The model under review builds one solid part; all positions refer to its coordinate system, in mm. Face numbers are marked on the shaded views. A direction names the side the tool comes from. Coordinates: 2 decimals unless noted, no trailing zeros. Write each loop counter-clockwise with the first axis right and the second up, starting at its lowest first coordinate (ties: lowest second). Pieces come first, ordered by that corner, then holes. Notation, with made-up numbers: M 19.5,49.5 L 38.5,49.5 A23 cw 38.5,88.5 Z; hole C 40.25,66.25 d11. An arc over 180 degrees is marked long. Answer as a JSON object with one key per item and string values.
```python
from build123d import *

# Parameters (mm, degrees)
BOSS_EXTRUDE1_DEPTH = 1013.2


with BuildPart() as part:
    # Sketch1 → Boss-Extrude1 (new body)
    with BuildSketch(Plane.XY):
        Polygon((1221.8, 1649.71), (2235, 1649.71), (2235, 0), (0, 0), (0, 1053.44), align=None)
        Polygon((2.5, 1051.878238321), (1222.377482381, 1647.21), (2232.5, 1647.21), (2232.5, 2.5), (2.5, 2.5), align=None, mode=Mode.SUBTRACT)
    extrude(amount=BOSS_EXTRUDE1_DEPTH)


solid = part.part
```
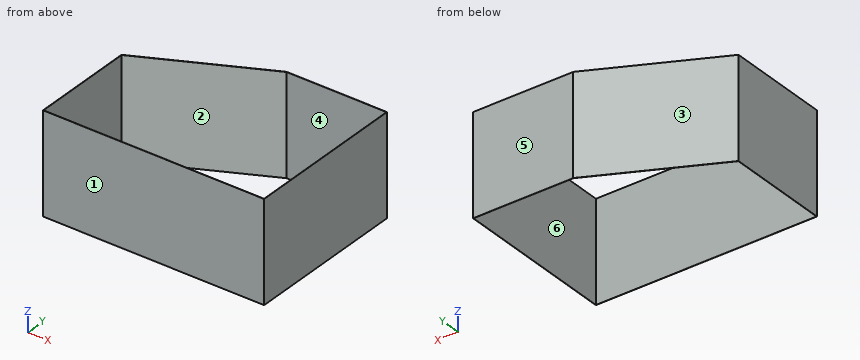
(1) Draft analysis for pull direction X (two halves, no side actions). For the marked faces 1, 2, 3 and 4, state which applies: released by +X, released by -X, zero draft, split by the parting line, or undercut.
Results list:
{"face 1": "zero draft", "face 2": "undercut", "face 3": "released by -X", "face 4": "undercut"}
(2) Add section C-C on z = 730. Give the boundary of the cut face in (x, y), and give its area (3 significant figures).
Results list:
{"outline": "M 0,0 L 2235,0 L 2235,1649.71 L 1221.8,1649.71 L 0,1053.44 Z; hole M 2.5,2.5 L 2232.5,2.5 L 2232.5,1647.21 L 1222.38,1647.21 L 2.5,1051.88 Z", "area": "18,300 mm²"}
(3) Add section A-A on x = 1362. Give the boundary of the cut face in (y, z).
Results list:
{"outline": "M 0,0 L 2.5,0 L 2.5,1013.2 L 0,1013.2 Z; M 1647.21,0 L 1649.71,0 L 1649.71,1013.2 L 1647.21,1013.2 Z"}
(4) For pin 1 Ø12 at (x, z) = (329, 668.5) entering from +Y; pin 2 Ø5 at (x, z) = (974, 269) entering from +Y; pin 3 Ø3 at (y, z) = (394, 376) entering from -X, all flat-tipped, find the tip position at first contact; note any pin that passes through.
Results list:
{"pin 1": "y = 1216.93", "pin 2": "y = 1530", "pin 3": "x = 0"}
(5) For the marked faces 5 and 6, list the 3-axis set-ups (+Z, -Z, +X, -X, +Y, -Y) from which the entire face can be reached by the end or side of a thin tool; tool diameter is ignored.
Results list:
{"face 5": "+Z, -Z, +X, -X, +Y", "face 6": "+Z, -Z"}
(6) Wall thickness on line 1 along X through (y, z) = (269.5, 859); line 2 along Y through (x, z) = (1358.5, 225.5); line 3 along X through (y, z) = (1155.5, 323): over which ranges is each line inside the solid? List them lowest first. Write a range as from..to.
Results list:
{"line 1": "0..2.5, 2232.5..2235", "line 2": "0..2.5, 1647.21..1649.71", "line 3": "209.13..214.83, 2232.5..2235"}
(7) Add section B-B on y = 797.5. Give the boundary of the cut face in (x, z), and give its area (3 significant figures).
Results list:
{"outline": "M 0,0 L 2.5,0 L 2.5,1013.2 L 0,1013.2 Z; M 2232.5,0 L 2235,0 L 2235,1013.2 L 2232.5,1013.2 Z", "area": "5,070 mm²"}
